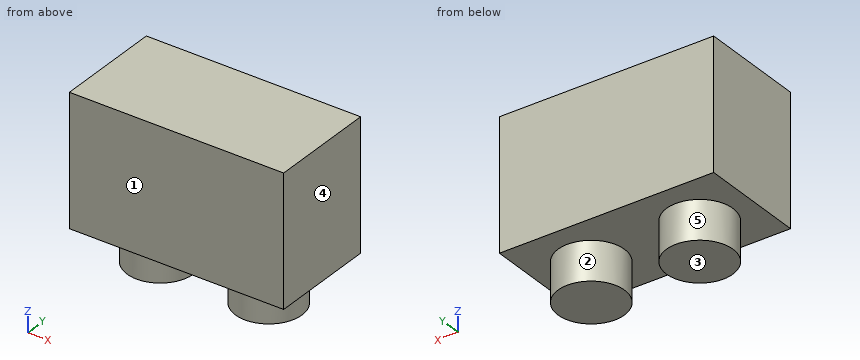
```python
from build123d import *

# Parameters (mm, degrees)
F0_W     = 15.7988
F0_H     = 7.8994
F0_R     = 2.44983
F1_DEPTH = 9.6012
F2_DEPTH = 2.8702


# Not quite as in the source:
# - a feature names something its author has since deleted; it is built from what else it names


with BuildPart() as f1:
    # F0 (on Top) → F1 (new body)
    with BuildSketch(Plane.XY):
        with Locations((-7.8994, -3.9497)):
            Rectangle(F0_W, F0_H)
        with Locations((-11.89863, -3.99923)):
            Circle(F0_R, mode=Mode.SUBTRACT)
        with Locations((-3.90017, -3.99923)):
            Circle(F0_R, mode=Mode.SUBTRACT)
        with Locations((-11.89863, -3.99923)):
            Circle(F0_R)
        with Locations((-3.90017, -3.99923)):
            Circle(F0_R)
    extrude(amount=F1_DEPTH)

    # F0 (on Top) → F2 (join)
    with BuildSketch(Plane.XY):
        with Locations((-3.90017, -3.99923)):
            Circle(F0_R)
        with Locations((-11.89863, -3.99923)):
            Circle(F0_R)
    extrude(amount=-F2_DEPTH)


solid = f1.part
```
Work out the finished part from the listing and answer in its coordinate system (mm). Face numbers are marked on the shaded views. A direction names the side the tool comes from. Round coordinates to 2 decimals unless told otherwise and drop trailing zeros. Write each loop counter-clockwise with the first axis right and the second up, starting at its lowest first coordinate (ties: lowest second). Pieces come first, ordered by that corner, then holes.
1) Consider probe 1 along Z at (x, y) = (-13, -6.25); probe 2 along Y at (x, z) = (-10.25, -0.5). Determine where each line is inside the solid, lowest interval first.
2) A cutting plane is placed at B-B on y = -5. Determine the outline of the cut face in (x, z), and give its area (3 significant figures).
3) Determine the mould class of the marked faces 3, 4 and 5 for opening direction X: pulls with the +X half, pulls with the -X half, needs draft (parallel to the pull), parting line crosses it, or undercut.
4) Which of the six approach directions +Z, -Z, +X, -X, +Y, -Y give full straight-line access (tool end or side, diameter ignored) to the marked faces 1 and 2?
5) A cutting plane is placed at D-D on y = -3.75. Determine the outline of the cut face in (x, z).
6) A cutting plane is placed at C-C on x = -2.5. Determine the outline of the cut face in (y, z).
7) A cutting plane is placed at A-A on x = -5.5. Determine the outline of the cut face in (y, z).
Entries:
1. probe 1: z = 0 to 9.6
1. probe 2: y = -5.81 to -2.19
2. outline: (-15.8, 0) - (-14.13, 0) - (-14.13, -2.87) - (-9.66, -2.87) - (-9.66, 0) - (-6.14, 0) - (-6.14, -2.87) - (-1.66, -2.87) - (-1.66, 0) - (0, 0) - (0, 9.6) - (-15.8, 9.6) - close
2. area: 177 mm2
3. face 3: needs draft
3. face 4: pulls with the +X half
3. face 5: undercut
4. face 1: +Z, -Z, +X, -X, -Y
4. face 2: -Z
5. outline: (-15.8, 0) - (-14.34, 0) - (-14.34, -2.87) - (-9.46, -2.87) - (-9.46, 0) - (-6.34, 0) - (-6.34, -2.87) - (-1.46, -2.87) - (-1.46, 0) - (0, 0) - (0, 9.6) - (-15.8, 9.6) - close
6. outline: (-7.9, 0) - (-6.01, 0) - (-6.01, -2.87) - (-1.99, -2.87) - (-1.99, 0) - (0, 0) - (0, 9.6) - (-7.9, 9.6) - close
7. outline: (-7.9, 0) - (-5.85, 0) - (-5.85, -2.87) - (-2.14, -2.87) - (-2.14, 0) - (0, 0) - (0, 9.6) - (-7.9, 9.6) - close
